Source: CAD feature listing. Evaluate the final solid. Frame: model axes, mm. A direction names the side the tool comes from. Round coordinates to 2 decimals unless told otherwise and drop trailing zeros. Loops run counter-clockwise (first coordinate to the right, second up) from the corner with the lowest first, then second, coordinate; pieces in that order, holes last. Notation, with made-up numbers: M 79,-27 L 100,-27 A25 cw 100,12 Z; hole C 34,24.5 d10. An arc over 180 degrees is marked long. One line per item, written item: value.
Autodesk Inventor part; units mm, degrees
ref_plane "YZ Plane" through (0, 0, 0) normal (1, 0, 0) x (0, 1, 0)
ref_plane "XZ Plane" through (0, 0, 0) normal (0, 1, 0) x (-1, 0, 0)
ref_plane "XY Plane" through (0, 0, 0) normal (0, 0, 1) x (1, 0, 0)
sketch "スケッチ1" plane through (0, 0, 0) normal (1, 0, 0) x (0, 1, 0)
  line L0 (-144.8102, -220.9081) -> (-144.8102, 234.0919)
  line L1 (-144.8102, -220.9081) -> (145.1898, -220.9081)
  line L2 (145.1898, -220.9081) -> (145.1898, -205.9081)
  line L3 (145.1898, -205.9081) -> (-144.8102, -205.9081)
  line L4 (-144.8102, -205.9081) -> (-144.8102, -220.9081)
  line L5 (145.1898, 234.0919) -> (145.1898, -220.9081)
  line L6 (145.1898, -220.9081) -> (160.1898, -220.9081)
  line L7 (160.1898, 234.0919) -> (160.1898, -220.9081)
  line L8 (0.1898, -205.9081) -> (0.1898, -220.9081)
  line L9 (125.1898, -205.9081) -> (125.1898, -220.9081)
  line L10 (145.1898, -198.4081) -> (160.1898, -198.4081)
  circle A0 centre (130.1898, -213.4081) radius 1.7
  circle A1 centre (140.1898, -213.4081) radius 1.7
  circle A2 centre (152.6898, -213.4081) radius 1.7
  circle A3 centre (152.6898, -203.4081) radius 1.7
  point P0 (0, 0)
  point P1 (-54.8102, -185.9081)
  point P2 (-152.3102, -203.4081)
  point P3 (-152.3102, -213.4081)
  point P4 (-139.8102, -213.4081)
  point P5 (-129.8102, -213.4081)
  dimension "d0" = 15
  dimension "d1" = 0
  dimension "d2" = 10
  dimension "d3" = 7.5
  dimension "d4" = 10
  dimension "d5" = 5
  dimension "d6" = 7.5
  dimension "d7" = 7.5
  dimension "d8" = 7.5
  dimension "d9" = 7.5
  dimension "d10" = 5
  dimension "d11" = 5
  dimension "d12" = 3.4
  dimension "d13" = 3.4
  dimension "d14" = 3.4
  dimension "d15" = 3.4
extrude "押し出し1" add sketch "スケッチ1" along normal blind 5 contours L9 L3 L2 L1 | L2 L5 L10 L7 L6
fillet "フィレット1" radius 2 6 edges at (2.5, 160.1898, -220.9081) (2.5, 160.1898, -198.4081) (2.5, 145.1898, -198.4081) (2.5, 145.1898, -205.9081) (2.5, 125.1898, -205.9081) (2.5, 125.1898, -220.9081)
properties part number "ball_loading_v1_Plate_ASP_F_3" material "ABS プラスチック"
1. Pin query (flat end, axial travel): pin 1 (3 mm diameter, centred on x = 1.5, z = -203, fed in from -Y); pin 2 (3 mm diameter, centred on x = 3.5, y = 131.5, fed in from +Z). Return the tip coordinate at first contact, or that it passes through.
Report:
pin 1: stops at y = 145.1
pin 2: stops at z = -205.91
2. Section query B-B (x = 3.3). Return the cut outline in (y, z), and give its area (3 significant figures).
Report:
outline: M 125.19,-218.91 A2 ccw 127.19,-220.91 L 158.19,-220.91 A2 ccw 160.19,-218.91 L 160.19,-200.41 A2 ccw 158.19,-198.41 L 147.19,-198.41 A2 ccw 145.19,-200.41 L 145.19,-203.91 A2 cw 143.19,-205.91 L 127.19,-205.91 A2 ccw 125.19,-207.91 Z; hole C 130.19,-213.41 d3.4; hole C 140.19,-213.41 d3.4; hole C 152.69,-213.41 d3.4; hole C 152.69,-203.41 d3.4
area: 598 mm2
3. Reachability of faces 1 (the face through (2.535, 125.76, -220.307)), 2 (the face through (2, 145.19, -202)) from +Z, -Z, +X, -X, +Y, -Y: full face, straight path, thin tool, end or side. Return the list, or none.
Report:
face 1: -Z, +X, -X, -Y
face 2: +Z, +X, -X, -Y
4. Section query A-A (z = -204.5). Return the cut outline in (x, y).
Report:
outline: M 0,145.1 L 5,145.1 L 5,151.39 L 0,151.39 Z; M 0,153.99 L 5,153.99 L 5,160.19 L 0,160.19 Z
5. Section query D-D (y = 136.5). Return the cut outline in (x, z).
Report:
outline: M 0,-220.91 L 5,-220.91 L 5,-205.91 L 0,-205.91 Z
6. Ray query, line 1 (Y direction, x = 0.9, z = -214); line 2 (Z direction, x = 0.85, y = 135.5); line 3 (Y direction, x = 1.7, z = -214.5). Return the intervals inside material, ascending. Write a range as [from, to].
Report:
line 1: y = [125.19, 128.6], [131.78, 138.6], [141.78, 151.1], [154.28, 160.19]
line 2: z = [-220.91, -205.91]
line 3: y = [125.19, 128.89], [131.49, 138.89], [141.49, 151.39], [153.99, 160.19]
7. Section query C-C (z = -212.75). Return the cut outline in (x, y).
Report:
outline: M 0,125.19 L 5,125.19 L 5,128.62 L 0,128.62 Z; M 0,131.76 L 5,131.76 L 5,138.62 L 0,138.62 Z; M 0,141.76 L 5,141.76 L 5,151.12 L 0,151.12 Z; M 0,154.26 L 5,154.26 L 5,160.19 L 0,160.19 Z
8. Pull-direction query (Y, two-part tool) for faces 3 (the face through (2.465, 130.974, -211.9)), 4 (the face through (2, 125.19, -213)), 5 (the face through (5, 146, -212)); classes: released by +Y, released by -Y, zero draft, split by the parting line, or undercut.
Report:
face 3: undercut
face 4: released by -Y
face 5: zero draft
